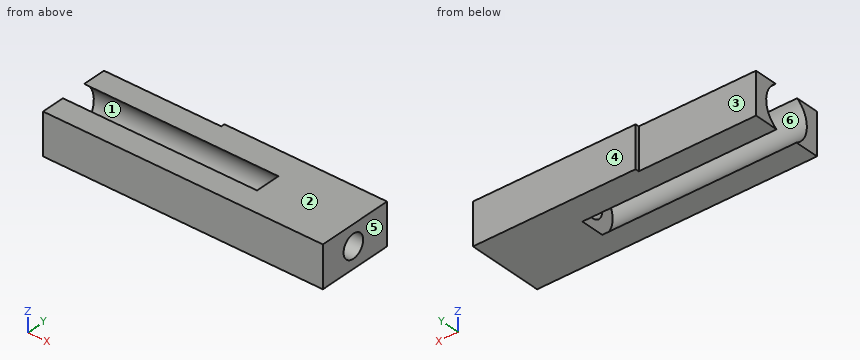
from build123d import *

# Parameters (mm, degrees)
CYLINDER001_R     = 2.8
CYLINDER001_DEPTH = 67.3
CYLINDER_R        = 5.8
CYLINDER_DEPTH    = 46.7
BOX001_W          = 28.2
BOX001_H          = 0.9
BOX001_DEPTH      = 10
BOX_W             = 67.3
BOX_H             = 18.3
BOX_DEPTH         = 10


with BuildPart() as cylinder001:
    # Cylinder001 → Cylinder001 (new body)
    with BuildSketch(Plane(origin=(0, 8.7, 5.06), x_dir=(0, 0, -1), z_dir=(1, 0, 0))):
        Circle(CYLINDER001_R)
    extrude(amount=CYLINDER001_DEPTH)


with BuildPart() as cylinder:
    # Cylinder → Cylinder (new body)
    with BuildSketch(Plane(origin=(0, 8.7, 5.06), x_dir=(0, 0, -1), z_dir=(1, 0, 0))):
        Circle(CYLINDER_R)
    extrude(amount=CYLINDER_DEPTH)


with BuildPart() as cube001:
    # Box001 → Box001 (new body)
    with BuildSketch(Plane(origin=(0, 17.4, 0), x_dir=(1, 0, 0), z_dir=(0, 0, 1))):
        with Locations((14.1, 0.45)):
            Rectangle(BOX001_W, BOX001_H)
    extrude(amount=BOX001_DEPTH)


with BuildPart() as cut002:
    # Box → Box (new body)
    with BuildSketch(Plane.XY):
        with Locations((33.65, 9.15)):
            Rectangle(BOX_W, BOX_H)
    extrude(amount=BOX_DEPTH)

    # Cut: cut Cube001
    add(cube001.part, mode=Mode.SUBTRACT)

    # Cut001: cut Cylinder
    add(cylinder.part, mode=Mode.SUBTRACT)

    # Cut002: cut Cylinder001
    add(cylinder001.part, mode=Mode.SUBTRACT)


solid = cut002.part
The listing builds one solid part. Answer for the finished solid, in the listing's coordinates (mm). Face numbers are marked on the shaded views. A direction names the side the tool comes from. Give positions to 0.01 mm unless a question says otherwise; leave off trailing zeros. Write each loop counter-clockwise with the first axis right and the second up, starting at its lowest first coordinate (ties: lowest second). Pieces come first, ordered by that corner, then holes. Notation, with made-up numbers: (13.25, -38.75) - (43.25, -38.75) arc R13 cw to (43.25, -22.75) - close; hole circle Ø5 at (84, 25.25). An arc over 180 degrees is marked (long way). Use a Markdown table: item, result.
1. Section C-C on x = 60.5 is taken. Write down the section's boundary in (y, z), plus the area to 3 significant figures.
Values follow:
| item | result |
|---|---|
| outline | (0, 0) - (18.3, 0) - (18.3, 10) - (0, 10) - close; hole circle Ø5.6 at (8.7, 5.06) |
| area | 158 mm² |
2. Section A-A on y = 8.7 is taken. Write down the section's boundary in (x, z).
Values follow:
| item | result |
|---|---|
| outline | (46.7, 0) - (67.3, 0) - (67.3, 2.26) - (46.7, 2.26) - close; (46.7, 7.86) - (67.3, 7.86) - (67.3, 10) - (46.7, 10) - close |
3. For a pull along Y with two mould halves and no side action, classify the marked faces 4, 5 and 6 as released by +Y, released by -Y, zero draft, split by the parting line, or undercut.
Values follow:
| item | result |
|---|---|
| face 4 | released by +Y |
| face 5 | zero draft |
| face 6 | undercut |
4. Each of these flat-tipped pins is pushed along its axis until it touches: P1, Ø1.5, axis at x = 22, z = 4.5, coming from the +Y side; P2, Ø1, axis at y = 18, z = 6.5, coming from the -X side; P3, Ø3, axis at y = 8, z = 6.5, coming from the -X side. Where does it stop, or does it pass through?
Values follow:
| item | result |
|---|---|
| P1 | stops at y = 17.4 |
| P2 | stops at x = 28.2 |
| P3 | stops at x = 46.7 |
5. Find the intervals of material crossed by probe 1 along Z at (x, y) = (62.25, 8.7); probe 2 along Y at (x, z) = (59.25, 5.06); probe 3 along X at (y, z) = (10.5, 8.25), in increasing order. Write a range as from..to.
Values follow:
| item | result |
|---|---|
| probe 1 | z = 0..2.26, 7.86..10 |
| probe 2 | y = 0..5.9, 11.5..18.3 |
| probe 3 | x = 46.7..67.3 |
6. A tool of negligible diameter and unlimited length cuts with its end or side. For the marked faces 1, 2 and 3, from which of +Z, -Z, +X, -X, +Y, -Y can it reach the whole face along a straight path? Write none if from no direction.
Values follow:
| item | result |
|---|---|
| face 1 | -X |
| face 2 | +Z, +X, -X, +Y, -Y |
| face 3 | +Z, -Z, -X, +Y |
7. Section D-D on x = 35.5 is taken. Write down the section's boundary in (y, z), plus the area to 3 significant figures.
Values follow:
| item | result |
|---|---|
| outline | (0, 0) - (5.87, 0) arc R5.8 cw to (5.66, 10) - (0, 10) - close; (11.53, 0) - (18.3, 0) - (18.3, 10) - (11.74, 10) arc R5.8 cw to start |
| area | 83.7 mm² |
8. Section B-B on z = 5.06 is taken. Write down the section's boundary in (x, y), plus the area to 3 significant figures.
Values follow:
| item | result |
|---|---|
| outline | (0, 0) - (67.3, 0) - (67.3, 5.9) - (46.7, 5.9) - (46.7, 2.9) - (0, 2.9) - close; (0, 14.5) - (46.7, 14.5) - (46.7, 11.5) - (67.3, 11.5) - (67.3, 18.3) - (28.2, 18.3) - (28.2, 17.4) - (0, 17.4) - close |
| area | 549 mm² |
